Geometry check sheet. Reference: drawing and pictorial views, mm from the part's lowest x, y, z. Round coordinates to 2 decimals unless told otherwise and drop trailing zeros. Order: outer loops, then holes, each group sorted by start corner. A loop starts at its lowest first (then second) coordinate and runs counter-clockwise, first axis right, second up.
(1) Thickness scan on L1, parallel to Y at x = 12.7, z = 0.8; L2, parallel to Y at x = 6, z = 0.45; L3, parallel to X at y = 7.75, z = 1.2. Record the ranges inside material, lowest first.
(2) Cross-section at B-B on x = 20.5. Enter the section's corners in (y, z).
(3) Cross-section at A-A on z = 0.4. Enter the section's corners in (x, y).
(4) Cross-section at C-C on y = 15.25. Enter the section's corners in (x, z), and give its area (3 significant figures).
(5) Gauge pin test, flat ends, axial feed: P1, Ø8, axis at x = 19.5, y = 18, coming from the -Z side; P2, Ø0.6, axis at x = 22, z = 0.5, coming from the +Y side; P3, Ø0.6, axis at x = 20.5, z = 0.5, coming from the -Y side. Record the tip position at first contact, or that the pin passes through.
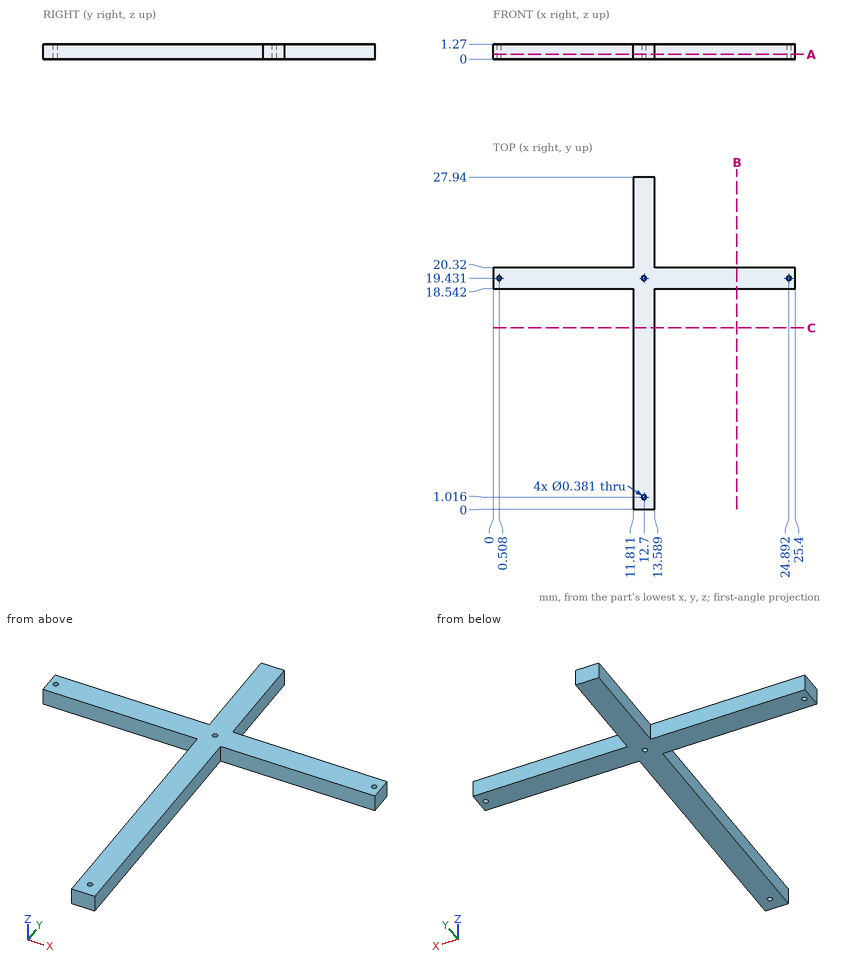
Found:
1. L1: y = 0 to 0.83, 1.21 to 19.24, 19.62 to 27.94
1. L2: y = 18.54 to 20.32
1. L3: x = 11.81 to 13.59
2. outline: (18.54, 0) - (20.32, 0) - (20.32, 1.27) - (18.54, 1.27) - close
3. outline: (0, 18.54) - (11.81, 18.54) - (11.81, 0) - (13.59, 0) - (13.59, 18.54) - (25.4, 18.54) - (25.4, 20.32) - (13.59, 20.32) - (13.59, 27.94) - (11.81, 27.94) - (11.81, 20.32) - (0, 20.32) - close; hole circle Ø0.38 at (0.51, 19.43); hole circle Ø0.38 at (12.7, 1.02); hole circle Ø0.38 at (12.7, 19.43); hole circle Ø0.38 at (24.89, 19.43)
4. outline: (11.81, 0) - (13.59, 0) - (13.59, 1.27) - (11.81, 1.27) - close
4. area: 2.26 mm2
5. P1: stops at z = 0
5. P2: stops at y = 20.32
5. P3: stops at y = 18.54
